```python
from build123d import *

# Parameters (mm, degrees)
SKETCH_3_R             = 50
EXTRUDE_2_DEPTH        = 20
CUT_EXTRUDE_2_DEPTH    = 74.484692283
PATTERN_LINEAR_2_DEPTH = 20


# Read off the part's stored shape, not the designer's step: 阵列(线性)2
with BuildPart() as part:
    # 草图3 → 凸台-拉伸2 (new body)
    with BuildSketch(Plane(origin=(0, 0, 0), x_dir=(1, 0, 0), z_dir=(0, 1, 0))):
        with Locations(Location((0, 0, 0), (0, 0, 270))):
            Circle(SKETCH_3_R)
    extrude(amount=EXTRUDE_2_DEPTH)

    # 草图4 → 切除-拉伸2 (cut, through all)
    with BuildSketch(Plane(origin=(0, 20, 0), x_dir=(1, 0, 0), z_dir=(0, 1, 0))):
        with BuildLine():
            Line((-17.095320997, -38.5), (17.095320997, -38.5))
            ThreePointArc((17.095320997, -38.5), (18.595320997, -40), (17.095320997, -41.5))
            Line((17.095320997, -41.5), (-17.095320997, -41.5))
            ThreePointArc((-17.095320997, -41.5), (-18.595320997, -40), (-17.095320997, -38.5))
        make_face()
    extrude(amount=-CUT_EXTRUDE_2_DEPTH, mode=Mode.SUBTRACT)

    # 阵列(线性)2 outline → 阵列(线性)2 (cut)
    with BuildSketch(Plane(origin=(0, 0, 0), x_dir=(1, 0, 0), z_dir=(0, 1, 0))):
        with BuildLine():
            Line((17.095320997, 41.5), (-17.095320997, 41.5))
            ThreePointArc((-17.095320997, 41.5), (-18.595320997, 40), (-17.095320997, 38.5))
            Line((-17.095320997, 38.5), (17.095320997, 38.5))
            ThreePointArc((17.095320997, 38.5), (18.595320997, 40), (17.095320997, 41.5))
        make_face()
        with BuildLine():
            Line((31.5, 31.5), (-31.5, 31.5))
            ThreePointArc((-31.5, 31.5), (-33, 30), (-31.5, 28.5))
            Line((-31.5, 28.5), (31.5, 28.5))
            ThreePointArc((31.5, 28.5), (33, 30), (31.5, 31.5))
        make_face()
        with BuildLine():
            Line((38.629651823, 21.5), (-38.629651823, 21.5))
            ThreePointArc((-38.629651823, 21.5), (-40.129651823, 20), (-38.629651823, 18.5))
            Line((-38.629651823, 18.5), (38.629651823, 18.5))
            ThreePointArc((38.629651823, 18.5), (40.129651823, 20), (38.629651823, 21.5))
        make_face()
        with BuildLine():
            Line((42.334973721, 11.5), (-42.334973721, 11.5))
            ThreePointArc((-42.334973721, 11.5), (-43.834973721, 10), (-42.334973721, 8.5))
            Line((-42.334973721, 8.5), (42.334973721, 8.5))
            ThreePointArc((42.334973721, 8.5), (43.834973721, 10), (42.334973721, 11.5))
        make_face()
        with BuildLine():
            Line((43.5, 1.5), (-43.5, 1.5))
            ThreePointArc((-43.5, 1.5), (-45, 0), (-43.5, -1.5))
            Line((-43.5, -1.5), (43.5, -1.5))
            ThreePointArc((43.5, -1.5), (45, 0), (43.5, 1.5))
        make_face()
        with BuildLine():
            Line((42.334973721, -8.5), (-42.334973721, -8.5))
            ThreePointArc((-42.334973721, -8.5), (-43.834973721, -10), (-42.334973721, -11.5))
            Line((-42.334973721, -11.5), (42.334973721, -11.5))
            ThreePointArc((42.334973721, -11.5), (43.834973721, -10), (42.334973721, -8.5))
        make_face()
        with BuildLine():
            Line((38.629651823, -18.5), (-38.629651823, -18.5))
            ThreePointArc((-38.629651823, -18.5), (-40.129651823, -20), (-38.629651823, -21.5))
            Line((-38.629651823, -21.5), (38.629651823, -21.5))
            ThreePointArc((38.629651823, -21.5), (40.129651823, -20), (38.629651823, -18.5))
        make_face()
        with BuildLine():
            Line((31.5, -28.5), (-31.5, -28.5))
            ThreePointArc((-31.5, -28.5), (-33, -30), (-31.5, -31.5))
            Line((-31.5, -31.5), (31.5, -31.5))
            ThreePointArc((31.5, -31.5), (33, -30), (31.5, -28.5))
        make_face()
    extrude(amount=PATTERN_LINEAR_2_DEPTH, mode=Mode.SUBTRACT)


solid = part.part
```
Here's how the part is built. I have some questions about the finished solid (model axes, mm). A direction names the side the tool comes from. Coordinates: 2 decimals unless noted, no trailing zeros. Order: outer loops, then holes, each group sorted by start corner. A loop starts at its lowest first (then second) coordinate and runs counter-clockwise, first axis right, second up.
Item 1: I'm going to push flat-ended pins straight in: pin 1 Ø1.5 at (x, y) = (-13, 4) entering from +Z; pin 2 Ø1 at (y, z) = (16, -9.5) entering from +X; pin 3 Ø1.5 at (x, y) = (33.5, 11.5) entering from +Z. Where does each tip first touch, or does it pass through?
Response values:
pin 1: stops at z = 48.48
pin 2: stops at x = 49.18
pin 3: stops at z = 37.78
Item 2: I need wall thicknesses on probe 1 along Z at (x, y) = (-38.5, 9); probe 2 along Z at (x, y) = (37.5, 6.25); probe 3 along X at (y, z) = (18.5, 1). Which ranges of each line are inside material? Lowest first, please.
Response values:
probe 1: z = -31.9 to -21.5, -18.5 to -11.5, -8.5 to -1.5, 1.5 to 8.5, 11.5 to 18.5, 21.5 to 31.9
probe 2: z = -33.07 to -21.5, -18.5 to -11.5, -8.5 to -1.5, 1.5 to 8.5, 11.5 to 18.5, 21.5 to 33.07
probe 3: x = -49.99 to -44.62, 44.62 to 49.99
Item 3: If we section it at B-B, the plane x = 34.5: List the corners of the cut face in (y, z) for me, then the cut area to 3 significant figures.
Response values:
outline: (0, -36.19) - (20, -36.19) - (20, -21.5) - (0, -21.5) - close; (0, -18.5) - (20, -18.5) - (20, -11.5) - (0, -11.5) - close; (0, -8.5) - (20, -8.5) - (20, -1.5) - (0, -1.5) - close; (0, 1.5) - (20, 1.5) - (20, 8.5) - (0, 8.5) - close; (0, 11.5) - (20, 11.5) - (20, 18.5) - (0, 18.5) - close; (0, 21.5) - (20, 21.5) - (20, 36.19) - (0, 36.19) - close
area: 1,150 mm2
Item 4: Which directions (+Z, -Z, +X, -X, +Y, -Y) give clear straight access to the entire face, cutting with the end or side of a thin tool? Please do faces 5 (the face through (-33, 10, -30)), 6 (the face through (1, 0, -12)).
Response values:
face 5: +Y, -Y
face 6: +Z, -Z, +X, -X, -Y
Item 5: If we section it at D-D, the plane x = 0: Give the number of separate pieces and of enclosed holes in the cut face, then the cut area to 3 significant figures.
Response values:
separate pieces: 10
enclosed holes: 0
area: 1,460 mm2
Item 6: If we section it at A-A, the plane z = -30: List the corners of the cut face in (x, y) for me.
Response values:
outline: (-40, 0) - (-33, 0) - (-33, 20) - (-40, 20) - close; (33, 0) - (40, 0) - (40, 20) - (33, 20) - close
Item 7: Thinking about a two-plate mould opening in X: for faces 1 (the face through (15.02, 9.86, 47.69)), 2 (the face through (0, 10, -28.5)), 3 (the face through (-1, 10, -8.5)), 4 (the face through (1, 20, -12)), which applies, pulls with the +X half, pulls with the -X half, needs draft (parallel to the pull), parting line crosses it, or undercut?
Response values:
face 1: parting line crosses it
face 2: undercut
face 3: undercut
face 4: needs draft
Item 8: If we section it at C-C, the plane z = -40: List the corners of the cut face in (x, y) for me, then the cut area to 3 significant figures.
Response values:
outline: (-30, 0) - (-18.6, 0) - (-18.6, 20) - (-30, 20) - close; (18.6, 0) - (30, 0) - (30, 20) - (18.6, 20) - close
area: 456 mm2
